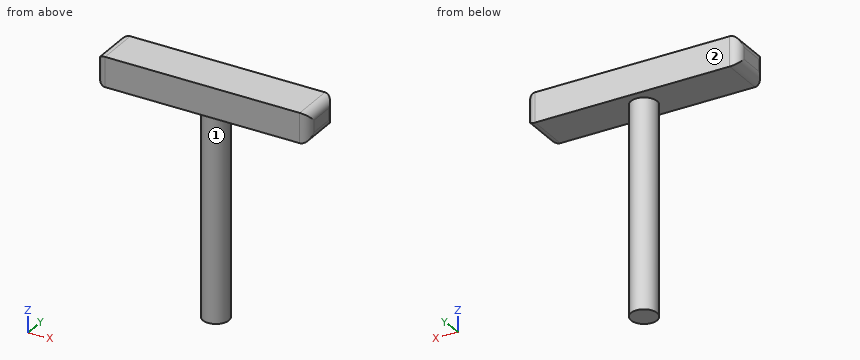
from build123d import *

# Parameters (mm, degrees)
F0_W     = 79.5655027032
F0_H     = 36.2267494202
F1_DEPTH = 12.7
F2_DEPTH = 12.7
F3_R     = 11.1269376105
F4_DEPTH = 177.8
F5_DEPTH = 50.8
F6_DEPTH = 50.8
F7_R     = 7.62
F8_R     = 7.62


with BuildPart() as f1:
    # F0 (on Top) → F1 (new body)
    with BuildSketch(Plane.XY):
        with Locations((-0.5556233227, -0.4444997758)):
            Rectangle(F0_W, F0_H)
    extrude(amount=F1_DEPTH)

    # F2 (add): a face of the model
    f2_faces = [f1.faces().sort_by_distance(p)[0] for p in [
        (-0.5556233227, -0.4444997758, 0),
    ]]
    extrude(f2_faces, amount=F2_DEPTH)

    # F3 (on face) → F4 (join)
    with BuildSketch(Plane(origin=(0, 0, -12.7), x_dir=(1, 0, 0), z_dir=(0, 0, -1))):
        Circle(F3_R)
    extrude(amount=F4_DEPTH)

    # F5 (add): a face of the model
    f5_faces = [f1.faces().sort_by_distance(p)[0] for p in [
        (-40.3383746743, -0.4444997758, 0),
    ]]
    extrude(f5_faces, amount=F5_DEPTH)

    # F6 (add): a face of the model
    f6_faces = [f1.faces().sort_by_distance(p)[0] for p in [
        (39.2271280289, -0.4444997758, 0),
    ]]
    extrude(f6_faces, amount=F6_DEPTH)

    # F7
    f7_edges = [f1.edges().sort_by_distance(p)[0] for p in [
        (90.027128, -0.4445, 12.7),
        (90.027128, 17.668875, 0),
        (90.027128, -0.4445, -12.7),
        (90.027128, -18.557874, 0),
    ]]
    fillet(f7_edges, radius=F7_R)

    # F8
    f8_edges = [f1.edges().sort_by_distance(p)[0] for p in [
        (-91.138375, 17.668875, 0),
        (-91.138375, -0.4445, 12.7),
        (-91.138375, -18.557874, 0),
        (-91.138375, -0.4445, -12.7),
    ]]
    fillet(f8_edges, radius=F8_R)


solid = f1.part
Read the model definition and answer for the solid it produces. Units are mm, in the model's axes. Face numbers are marked on the shaded views. A direction names the side the tool comes from. Give positions to 0.01 mm unless a question says otherwise; leave off trailing zeros. Loops run counter-clockwise (first coordinate to the right, second up) from the corner with the lowest first, then second, coordinate; pieces in that order, holes last. Notation, with made-up numbers: (75.25, 12.5) - (109.25, 12.5) arc R11 cw to (109.25, 33.5) - close; hole circle Ø9 at (56, 66). An arc over 180 degrees is marked (long way). Answer as CSV lines item,"result". Start each with the question number.
1) Find section C-C (z = -133.5). Write down the section's boundary in (x, y).
2) Each of these flat-tipped pins is pushed along its axis until it touches: pin 1 Ø1.5 at (y, z) = (-0.5, -116.5) entering from +X; pin 2 Ø2 at (y, z) = (7.5, -102) entering from +X; pin 3 Ø11 at (x, y) = (27, 1) entering from -Z. Where does it stop, or does it pass through?
3) Find section D-D (x = 34). Write down the section's boundary in (y, z).
4) Find section B-B (x = 0). Write down the section's boundary in (y, z).
5) Find section A-A (y = 0). Write down the section's boundary in (x, z), then the cut area to 3 significant figures.
6) Straight lines are drawn through the part: L1, parallel to Z at x = -71, y = 15; L2, parallel to X at y = 10.5, z = -5.5 (3 decimals); L3, parallel to X at y = -1, z = -34.5. For each, find the intervals that lie inside material, in ascending order. Write a range as from..to.
7) Which of the six approach directions +Z, -Z, +X, -X, +Y, -Y give full straight-line access (tool end or side, diameter ignored) to the marked faces 1 and 2?
Findings below:
1,outline,"circle Ø22.25 at (0, 0)"
2,pin 1,"x = 11.13"
2,pin 2,"x = 9.03"
2,pin 3,"z = -12.7"
3,outline,"(-18.56, -12.7) - (17.67, -12.7) - (17.67, 12.7) - (-18.56, 12.7) - close"
4,outline,"(-18.56, -12.7) - (-11.13, -12.7) - (-11.13, -190.5) - (11.13, -190.5) - (11.13, -12.7) - (17.67, -12.7) - (17.67, 12.7) - (-18.56, 12.7) - close"
5,outline,"(-91.14, -5.08) arc R7.62 ccw to (-83.52, -12.7) - (-11.13, -12.7) - (-11.13, -190.5) - (11.13, -190.5) - (11.13, -12.7) - (82.41, -12.7) arc R7.62 ccw to (90.03, -5.08) - (90.03, 5.08) arc R7.62 ccw to (82.41, 12.7) - (-83.52, 12.7) arc R7.62 ccw to (-91.14, 5.08) - close"
5,area,"8,510 mm^2"
6,L1,"-12.7..12.7"
6,L2,"-91.125..90.014"
6,L3,"-11.08..11.08"
7,face 1,"-Z"
7,face 2,"+Z, -Z, +X, -X, +Y"
